Part print with two shaded views. Sizes in mm from the minimum x, y, z corner. A direction names the side the tool comes from. Give positions to 0.01 mm unless a question says otherwise; leave off trailing zeros. Loops run counter-clockwise (first coordinate to the right, second up) from the corner with the lowest first, then second, coordinate; pieces in that order, holes last. Notation, with made-up numbers: M -18.5,44 L -10.5,44 A13 ccw -10.5,51 Z; hole C 3,-16.75 d5. An arc over 180 degrees is marked long. Answer as a JSON object with one key per item and string values. Group by question number.
1. Drop flat-ended pins along their axis: pin 1 Ø2.5 at (x, z) = (48.5, 9) entering from -Y; pin 2 Ø1.5 at (x, z) = (9.5, 11) entering from -Y; pin 3 Ø1 at (x, z) = (5.5, 10.5) entering from -Y. Give the stop position or say it passes through.
2. Slice it at B-B (z = 9). List the corners of the cut face in (x, y), then the cut area to 3 significant figures.
3. Slice it at A-A (y = 15). List the corners of the cut face in (x, z).
4. Slice it at C-C (x = 38). List the corners of the cut face in (y, z).
5. 3-axis set-ups, long thin cutter, end or side, ignore diameter. For the marked faces 4, 5 and 6: which of +Z, -Z, +X, -X, +Y, -Y reach the whole face in a straight line?
6. Mould opens along Z. For the marked faces 1, 2 and 3 say: released by +Z, released by -Z, zero draft, split by the parting line, or undercut.
7. Slice it at D-D (y = 9). List the corners of the cut face in (x, z), then the cut area to 3 significant figures.
8. Drill centre lines: line 1 along Z through (x, y) = (40.5, 10.25); line 2 along X through (y, z) = (6.25, 16.25); line 3 along Y through (x, z) = (60.5, 11.5). Where is each one in solid material? Low to high. Write a range as [from, to].
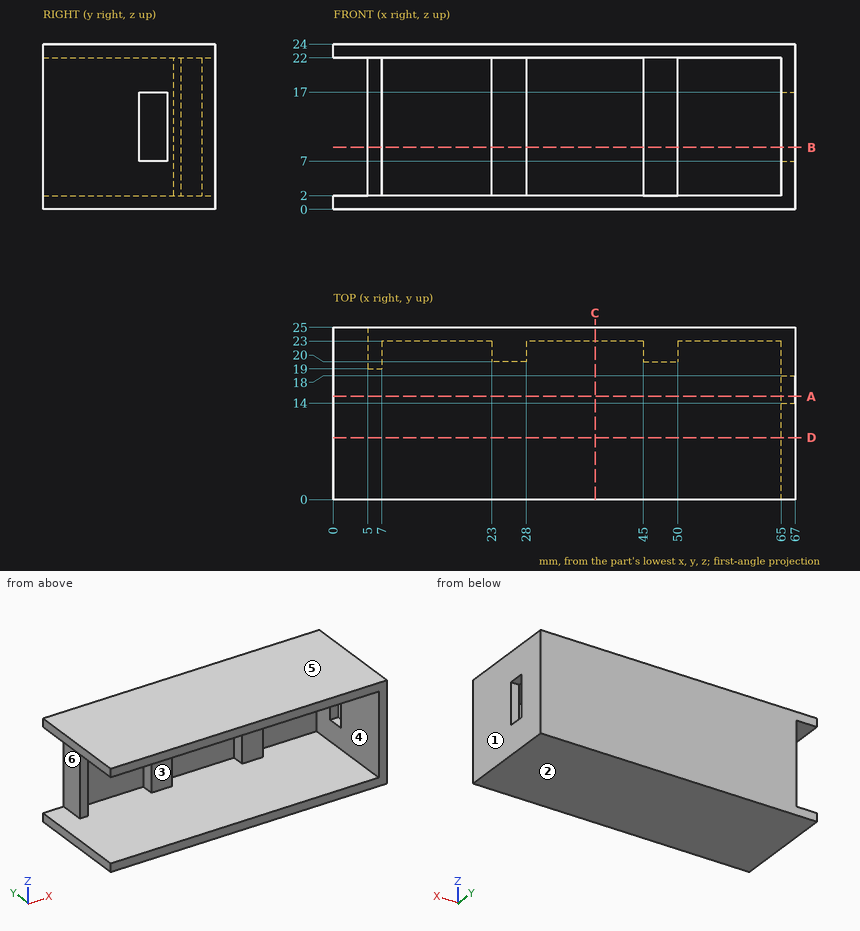
Established:
{
 "1": {"pin 1": "stops at y = 20", "pin 2": "stops at y = 23", "pin 3": "stops at y = 19"},
 "2": {"outline": "M 5,19 L 7,19 L 7,23 L 23,23 L 23,20 L 28,20 L 28,23 L 45,23 L 45,20 L 50,20 L 50,23 L 65,23 L 65,18 L 67,18 L 67,25 L 5,25 Z; M 65,0 L 67,0 L 67,14 L 65,14 Z", "area": "200 mm^2"},
 "3": {"outline": "M 0,0 L 67,0 L 67,7 L 65,7 L 65,2 L 0,2 Z; M 0,22 L 65,22 L 65,17 L 67,17 L 67,24 L 0,24 Z"},
 "4": {"outline": "M 0,0 L 25,0 L 25,24 L 0,24 L 0,22 L 23,22 L 23,2 L 0,2 Z"},
 "5": {"face 4": "-Y", "face 5": "+Z, +X, -X, +Y, -Y", "face 6": "-X, +Y, -Y"},
 "6": {"face 1": "zero draft", "face 2": "released by -Z", "face 3": "undercut"},
 "7": {"outline": "M 0,0 L 67,0 L 67,24 L 0,24 L 0,22 L 65,22 L 65,2 L 0,2 Z", "area": "308 mm^2"},
 "8": {"line 1": "z = [0, 2], [22, 24]", "line 2": "x = [65, 67]", "line 3": "y = [23, 25]"}
}
